Autodesk Inventor part; units mm, degrees
ref_plane "YZ Plane" through (0, 0, 0) normal (1, 0, 0) x (0, 1, 0)
ref_plane "XZ Plane" through (0, 0, 0) normal (0, 1, 0) x (-1, 0, 0)
ref_plane "XY Plane" through (0, 0, 0) normal (0, 0, 1) x (1, 0, 0)
sketch "Sketch1" plane through (0, 0, 0) normal (0, 1, 0) x (-1, 0, 0)
  line L0 (0, 0) -> (19.05, 0)
  line L1 (19.05, 0) -> (19.05, -38.1)
  line L2 (19.05, -38.1) -> (0, -38.1)
  line L3 (0, -38.1) -> (0, 0)
  line L4 (15.875, -34.925) -> (15.875, -3.175)
  line L5 (15.875, -3.175) -> (3.175, -3.175)
  line L6 (3.175, -3.175) -> (3.175, -34.925)
  line L7 (3.175, -34.925) -> (15.875, -34.925)
  dimension "d0" = 19.05
  dimension "d1" = 38.1
  dimension "d2" = 3.175
extrude "Extrusion1" add sketch "Sketch1" along normal blind 190.5
sketch "Sketch2" plane through (-19.05, 0, 0) normal (0, 0, 1) x (1, 0, 0)
  circle A0 centre (9.525, 177.8) radius 5
  line L0 (15.875, 0) -> (15.875, 190.5)
  line L1 (0, 0) -> (19.05, 0)
  line L2 (19.05, 0) -> (19.05, 190.5)
  line L3 (0, 190.5) -> (19.05, 190.5)
  line L4 (0, 0) -> (0, 190.5)
  point P0 (9.525, 190.5)
  dimension "d5" = 10
  dimension "d6" = 9.525
  dimension "d7" = 12.7
extrude "Extrusion2" cut sketch "Sketch2" against normal blind 204.7875 contours A0
sketch "Sketch3" plane through (0, 0, 0) normal (1, 0, 0) x (0, 0, -1)
  line L0 (25.3873, 190.5) -> (25.3873, 0)
  line L1 (38.1, 190.5) -> (38.1, 0)
  line L2 (38.1, 0) -> (0, 0)
  line L3 (38.1, 190.5) -> (25.3873, 190.5)
  line L4 (38.1, 0) -> (38.1, 190.5)
  line L5 (25.3873, 190.5) -> (38.1, 190.5)
  line L6 (38.1, 190.5) -> (0, 190.5)
  line L7 (0, 190.5) -> (38.1, 190.5)
  line L8 (12.6873, 190.5) -> (12.6873, 0)
  circle A0 centre (25.3873, 19.05) radius 5
  circle A1 centre (12.6873, 44.45) radius 5
  circle A2 centre (25.3873, 69.85) radius 5
  circle A3 centre (25.3873, 120.65) radius 5
  circle A4 centre (12.6873, 95.25) radius 5
  circle A5 centre (12.6873, 146.05) radius 5
  dimension "d10" = 12.7
  dimension "d11" = 10
  dimension "d12" = 10
  dimension "d15" = 50.8
  dimension "d20" = 19.05
  dimension "d21" = 25.4
  dimension "d24" = 50.8
extrude "Extrusion3" cut sketch "Sketch3" against normal blind 204.7875 contours A3 L0 | L0 A3 | A5 L8 | L8 A5 | A2 L0 | L0 A2 | A0 L0 | L0 A0 | A4 L8 | L8 A4 | A1 L8 | L8 A1
properties part number "hinge base"
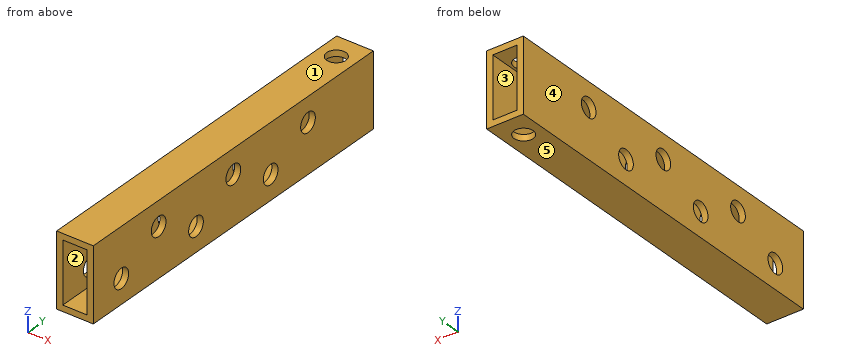
Can you work these out from the model? Positions are in its coordinate system, mm. Face numbers are marked on the shaded views. A direction names the side the tool comes from. Coordinates: 2 decimals unless noted, no trailing zeros. Loops run counter-clockwise (first coordinate to the right, second up) from the corner with the lowest first, then second, coordinate; pieces in that order, holes last. Notation, with made-up numbers: (-30.75, 81.5) -> (26.25, 81.5) arc R12 ccw to (26.25, 86.5) -> close; hole circle Ø10 at (-11, 37). An arc over 180 degrees is marked (long way). Answer as a JSON object with one key per item and string values.
1) Imagine slicing it at C-C (y = 177.8). Please give me the cut outline in (x, z) (3 decimals), then the cut area to 3 significant figures.
Results:
{"outline": "(-19.05, -38.1) -> (-14.525, -38.1) -> (-14.525, -34.925) -> (-15.875, -34.925) -> (-15.875, -3.175) -> (-14.525, -3.175) -> (-14.525, 0) -> (-19.05, 0) -> close; (-4.525, -38.1) -> (0, -38.1) -> (0, 0) -> (-4.525, 0) -> (-4.525, -3.175) -> (-3.175, -3.175) -> (-3.175, -34.925) -> (-4.525, -34.925) -> close", "area": "259 mm^2"}
2) Imagine slicing it at D-D (x = -12). Please give me the cut outline in (y, z) (3 decimals).
Results:
{"outline": "(0, -38.1) -> (173.456, -38.1) -> (173.456, -34.925) -> (0, -34.925) -> close; (0, -3.175) -> (173.456, -3.175) -> (173.456, 0) -> (0, 0) -> close; (182.144, -38.1) -> (190.5, -38.1) -> (190.5, -34.925) -> (182.144, -34.925) -> close; (182.144, -3.175) -> (190.5, -3.175) -> (190.5, 0) -> (182.144, 0) -> close"}
3) Imagine slicing it at A-A (y = 137). Please give me the cut outline in (x, z) (3 decimals).
Results:
{"outline": "(-19.05, -38.1) -> (0, -38.1) -> (0, 0) -> (-19.05, 0) -> close; hole (-15.875, -34.925) -> (-3.175, -34.925) -> (-3.175, -3.175) -> (-15.875, -3.175) -> close"}
4) Imagine slicing it at B-B (z = -5.5). Please give me the cut outline in (x, y) (3 decimals), then the cut area to 3 significant figures.
Results:
{"outline": "(-19.05, 0) -> (-15.875, 0) -> (-15.875, 190.5) -> (-19.05, 190.5) -> close; (-3.175, 0) -> (0, 0) -> (0, 190.5) -> (-3.175, 190.5) -> close", "area": "1,210 mm^2"}
5) For the marked faces 1 and 2, which set-ups out of +Z, -Z, +X, -X, +Y, -Y let a thin tool reach every point of the face, with its end or its side?
Results:
{"face 1": "+Z, +X, -X, +Y, -Y", "face 2": "+Y, -Y"}
6) If I drill on line 1 (Y direction, x = -18, z = -13); line 2 (X direction, y = 73, z = -30) (3 decimals); line 3 (Z direction, x = -7.25, y = 11.5) (3 decimals), over which ranges is the centre line in solid material (lowest first)?
Results:
{"line 1": "y = 0 to 39.46, 49.44 to 90.26, 100.24 to 141.06, 151.04 to 190.5", "line 2": "x = -19.05 to -15.875, -3.175 to 0", "line 3": "z = -38.1 to -34.925, -3.175 to 0"}
7) Thinking about a two-plate mould opening in Z: for the marked faces 3, 4 and 5, which applies, pulls with the +Z half, pulls with the -Z half, needs draft (parallel to the pull), parting line crosses it, or undercut?
Results:
{"face 3": "undercut", "face 4": "needs draft", "face 5": "pulls with the -Z half"}
